Geometry: final body of the model. Coordinates: model frame, mm. Face numbers are marked on the shaded views. A direction names the side the tool comes from. Give positions to 0.01 mm unless a question says otherwise; leave off trailing zeros. Write each loop counter-clockwise with the first axis right and the second up, starting at its lowest first coordinate (ties: lowest second). Pieces come first, ordered by that corner, then holes. Notation, with made-up numbers: (41.5, 51) -> (45.5, 51) arc R27 cw to (45.5, 72) -> close; hole circle Ø1 at (-28, 47.5). An arc over 180 degrees is marked (long way). Answer in a Markdown table with one row per item. Add a question column.
Item 1: Section query D-D on y = 3.5. Output: boundary loops of the cut face in (x, z).
Item 2: Access query for the marked faces 1, 2 and 3. Directions: +Z, -Z, +X, -X, +Y, -Y. A direction counts if a zero-diameter tool reaches every point of the face in a straight line with its end or side. Return the directions, or none.
Item 3: Section query B-B on z = -38. Output: boundary loops of the cut face in (x, y), plus the area to 3 significant figures.
Item 4: First-contact query: P1, Ø6, axis at x = 38.5, y = 7.5, coming from the +Z side; P2, Ø12, axis at x = 10, z = -25, coming from the +Y side; P3, Ø2, axis at y = 7, z = -3, coming from the +X side; P4, Ø4.5, axis at x = -3, y = 5.5, coming from the -Z side. Flat tips, straight axial feed; report the tip coordinate or a pass-through.
Item 5: Section query A-A on y = 7. Output: boundary loops of the cut face in (x, z), plus the area to 3 significant figures.
Item 6: Material intervals for probe 1 along Y at (x, z) = (74, -38); probe 2 along X at (y, z) = (6.5, -32); probe 3 along Z at (x, y) = (-3, 12.25), sorted ascending. Write a range as from..to.
Item 7: Section query C-C on x = 1. Output: boundary loops of the cut face in (y, z), plus the area to 3 significant figures.
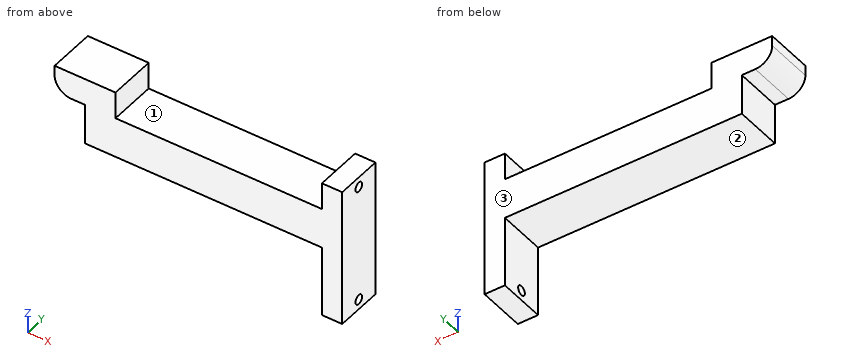
Autodesk Inventor part; units mm, degrees
ref_plane "YZ Plane" through (0, 0, 0) normal (1, 0, 0) x (0, 1, 0)
ref_plane "XZ Plane" through (0, 0, 0) normal (0, 1, 0) x (-1, 0, 0)
ref_plane "XY Plane" through (0, 0, 0) normal (0, 0, 1) x (1, 0, 0)
sketch "Sketch1" plane through (0, 0, 0) normal (1, 0, 0) x (0, 1, 0)
  line L0 (0, 0) -> (14, 0)
  line L1 (14, 0) -> (14, -20)
  line L2 (14, -20) -> (0, -20)
  line L3 (0, -20) -> (0, 0)
  line L4 (14, -20) -> (0, -20)
  line L5 (0, -20) -> (0, -20)
  line L6 (0, -20) -> (14, -20)
  line L7 (14, -20) -> (14, -20)
  line L8 (0, 0) -> (0, -8)
  line L9 (0, -8) -> (14, -8)
  line L10 (14, -8) -> (14, 0)
  point P0 (14, -8)
  dimension "d12" = 14
  dimension "d13" = 20
  dimension "d14" = 12
  dimension "d15" = 0
extrude "Extrusion6" add sketch "Sketch1" along normal blind 70 contours L9 L1 L2 L3
extrude "Extrusion7" add sketch "Sketch1" against normal mid plane 18 contours L0 L1 L9 L3
fillet "Fillet1" radius 5 1 edges at (-9, 7, -8)
sketch "Sketch6" plane through (70, 0, 0) normal (1, 0, 0) x (0, 0, -1)
  line L0 (8, 14) -> (0, 14)
  line L1 (0, 14) -> (41, 14)
  line L2 (41, 14) -> (41, 0)
  line L3 (41, 0) -> (0, 0)
  line L4 (0, 0) -> (0, 14)
  circle A0 centre (38, 7) radius 1.4
  circle A1 centre (3, 7) radius 1.4
  line L5 (8, 14) -> (8, 0)
  dimension "d21" = 41
  dimension "d22" = 2.8
  dimension "d23" = 3
  dimension "d24" = 2.8
  dimension "d25" = 35
  dimension "d26" = 5
extrude "Extrusion8" add sketch "Sketch6" along normal blind 6
properties part number "_3DPrint"
Findings below:
| question | item | result |
|---|---|---|
| 1 | outline | (-9, -3) arc R5 ccw to (-4, -8) -> (0, -8) -> (0, -20) -> (70, -20) -> (70, -41) -> (76, -41) -> (76, 0) -> (70, 0) -> (70, -8) -> (9, -8) -> (9, 0) -> (-9, 0) -> close |
| 2 | face 1 | +Z, +Y, -Y |
| 2 | face 2 | -Z, -X, +Y, -Y |
| 2 | face 3 | +Z, -Z, +X, -X, +Y |
| 3 | outline | (70, 0) -> (76, 0) -> (76, 5.6) -> (70, 5.6) -> close; (70, 8.4) -> (76, 8.4) -> (76, 14) -> (70, 14) -> close |
| 3 | area | 67.2 mm^2 |
| 4 | P1 | stops at z = -8 |
| 4 | P2 | stops at y = 14 |
| 4 | P3 | stops at x = 9 |
| 4 | P4 | stops at z = -8 |
| 5 | outline | (-9, -3) arc R5 ccw to (-4, -8) -> (0, -8) -> (0, -20) -> (70, -20) -> (70, -36.6) -> (76, -36.6) -> (76, -4.4) -> (70, -4.4) -> (70, -8) -> (9, -8) -> (9, 0) -> (-9, 0) -> close; (70, -41) -> (76, -41) -> (76, -39.4) -> (70, -39.4) -> close; (70, -1.6) -> (76, -1.6) -> (76, 0) -> (70, 0) -> close |
| 5 | area | 1,190 mm^2 |
| 6 | probe 1 | y = 0..5.6, 8.4..14 |
| 6 | probe 2 | x = 70..76 |
| 6 | probe 3 | z = -8..0 |
| 7 | outline | (0, -20) -> (14, -20) -> (14, 0) -> (0, 0) -> close |
| 7 | area | 280 mm^2 |
